Source: CAD feature listing. Evaluate the final solid. Frame: model axes, mm. Face numbers are marked on the shaded views. Give positions to 0.01 mm unless a question says otherwise; leave off trailing zeros. Loops run counter-clockwise (first coordinate to the right, second up) from the corner with the lowest first, then second, coordinate; pieces in that order, holes last.
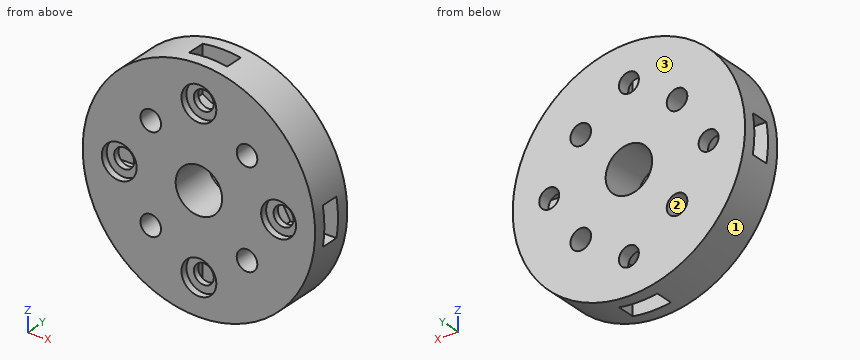
```python
from build123d import *

# Parameters (mm, degrees)
SKETCH1_R                      = 6.05
SKETCH1_R_2                    = 3.05
BOSS_EXTRUDE1_DEPTH            = 10
SKETCH2_R                      = 17.5
BOSS_EXTRUDE2_DEPTH            = 6.5
CUT_EXTRUDE1_REACH             = 28.693
SKETCH3_R                      = 1.5
CUT_EXTRUDE2_DEPTH             = 30.744747435
CUT_EXTRUDE2_DEPTH_BACK        = 30.744747435
SKETCH4_R                      = 1.5
CUT_EXTRUDE3_REACH             = 28.693
SKETCH6_R                      = 3.5
CUT_EXTRUDE3_DIRECTION_2_REACH = 28.693
SKETCH8_W                      = 5.75
SKETCH8_H                      = 2.75
CUT_EXTRUDE4_DEPTH             = 5
CUT_EXTRUDE5_DEPTH             = 2.75
CIRPATTERN1_START              = 11.875
CIRPATTERN1_OUTLINE_R          = 1.5
CIRPATTERN1_DEPTH              = 2.75
SKETCH10_R                     = 6.05
CUT_EXTRUDE6_DEPTH             = 10
SKETCH11_R                     = 1.55
CUT_EXTRUDE7_DEPTH             = 10
SKETCH12_R                     = 2.625
CUT_EXTRUDE8_DEPTH             = 1
CIRPATTERN2_COUNT              = 4


# Read off the part's stored shape, not the designer's step: CirPattern1
with BuildPart() as part:
    # Sketch1 → Boss-Extrude1 (new body)
    with BuildSketch(Plane(origin=(0, 0, 0), x_dir=(1, 0, 0), z_dir=(0, 1, 0))):
        with Locations(Location((0, 0, 0), (0, 0, 270))):
            Circle(SKETCH1_R)
        with Locations(Location((0, 0, 0), (0, 0, 270))):
            Circle(SKETCH1_R_2, mode=Mode.SUBTRACT)
    extrude(amount=BOSS_EXTRUDE1_DEPTH)

    # Sketch2 → Boss-Extrude2 (add)
    with BuildSketch(Plane(origin=(0, 10, 0), x_dir=(1, 0, 0), z_dir=(0, 1, 0))):
        with Locations(Location((0, 0, 0), (0, 0, 90))):
            Circle(SKETCH2_R)
    extrude(amount=BOSS_EXTRUDE2_DEPTH)

    # Sketch3 → Cut-Extrude1 (cut, up to next)
    with BuildSketch(Plane.XZ.offset(-10), mode=Mode.PRIVATE) as cut_extrude1_sk1:
        with Locations(Location((12, 0, 0), (0, 0, 270))):
            Circle(SKETCH3_R)
    cut_extrude1_tool1 = extrude(cut_extrude1_sk1.sketch, amount=-CUT_EXTRUDE1_REACH, mode=Mode.PRIVATE) & part.part
    # Sketch3 → Cut-Extrude1 (cut, up to next)
    with BuildSketch(Plane.XZ.offset(-10), mode=Mode.PRIVATE) as cut_extrude1_sk2:
        with Locations(Location((0, -12, 0), (0, 0, 270))):
            Circle(SKETCH3_R)
    cut_extrude1_tool2 = extrude(cut_extrude1_sk2.sketch, amount=-CUT_EXTRUDE1_REACH, mode=Mode.PRIVATE) & part.part
    # Sketch3 → Cut-Extrude1 (cut, up to next)
    with BuildSketch(Plane.XZ.offset(-10), mode=Mode.PRIVATE) as cut_extrude1_sk3:
        with Locations(Location((-12, 0, 0), (0, 0, 270))):
            Circle(SKETCH3_R)
    cut_extrude1_tool3 = extrude(cut_extrude1_sk3.sketch, amount=-CUT_EXTRUDE1_REACH, mode=Mode.PRIVATE) & part.part
    # Sketch3 → Cut-Extrude1 (cut, up to next)
    with BuildSketch(Plane.XZ.offset(-10), mode=Mode.PRIVATE) as cut_extrude1_sk4:
        with Locations(Location((0, 12, 0), (0, 0, 270))):
            Circle(SKETCH3_R)
    cut_extrude1_tool4 = extrude(cut_extrude1_sk4.sketch, amount=-CUT_EXTRUDE1_REACH, mode=Mode.PRIVATE) & part.part
    add(cut_extrude1_tool1.solids().sort_by_distance((12, 10, 0))[0], mode=Mode.SUBTRACT)
    add(cut_extrude1_tool2.solids().sort_by_distance((0, 10, -12))[0], mode=Mode.SUBTRACT)
    add(cut_extrude1_tool3.solids().sort_by_distance((-12, 10, 0))[0], mode=Mode.SUBTRACT)
    add(cut_extrude1_tool4.solids().sort_by_distance((0, 10, 12))[0], mode=Mode.SUBTRACT)

    # Sketch4 → Cut-Extrude2 (cut, two sides: drawn at the far end of the back side and taken through both)
    with BuildSketch(Plane.XY.offset(-CUT_EXTRUDE2_DEPTH_BACK)):
        with Locations((0, 4.916404418)):
            Circle(SKETCH4_R)
    extrude(amount=CUT_EXTRUDE2_DEPTH + CUT_EXTRUDE2_DEPTH_BACK, mode=Mode.SUBTRACT)

    # Sketch6 → Cut-Extrude3 (cut, up to next)
    with BuildSketch(Plane(origin=(0, 10, 0), x_dir=(-1, 0, 0), z_dir=(0, -1, 0)), mode=Mode.PRIVATE) as cut_extrude3_sk1:
        with Locations(Location((0, 0, 0), (0, 0, 270))):
            Circle(SKETCH6_R)
    cut_extrude3_tool1 = extrude(cut_extrude3_sk1.sketch, amount=-CUT_EXTRUDE3_REACH, mode=Mode.PRIVATE) & part.part
    add(cut_extrude3_tool1.solids().sort_by_distance((0, 10, 0))[0], mode=Mode.SUBTRACT)

    # Sketch6 → Cut-Extrude3 direction 2 (cut, up to next)
    with BuildSketch(Plane(origin=(0, 10, 0), x_dir=(-1, 0, 0), z_dir=(0, -1, 0)), mode=Mode.PRIVATE) as cut_extrude3_direction_2_sk1:
        with Locations(Location((0, 0, 0), (0, 0, 270))):
            Circle(SKETCH6_R)
    cut_extrude3_direction_2_tool1 = extrude(cut_extrude3_direction_2_sk1.sketch, amount=CUT_EXTRUDE3_DIRECTION_2_REACH, mode=Mode.PRIVATE) & part.part
    add(cut_extrude3_direction_2_tool1.solids().sort_by_distance((0, 10, 0))[0], mode=Mode.SUBTRACT)

    # Sketch8 → Cut-Extrude4 (cut)
    with BuildSketch(Plane(origin=(17.5, 0, 0), x_dir=(0, 0, -1), z_dir=(1, 0, 0))):
        with Locations((0, 13.25)):
            Rectangle(SKETCH8_W, SKETCH8_H)
    extrude(amount=-CUT_EXTRUDE4_DEPTH, mode=Mode.SUBTRACT)

    # Sketch9 → Cut-Extrude5 (cut)
    with BuildSketch(Plane.XZ.offset(-14.625)):
        Polygon((15.319764048, 0), (13.659882024, 2.875), (10.340117976, 2.875), (8.680235952, 0), (10.340117976, -2.875), (13.659882024, -2.875), align=None)
    extrude(amount=CUT_EXTRUDE5_DEPTH, mode=Mode.SUBTRACT)

    # CirPattern1 outline → CirPattern1 (cut)
    # profile 1 of 3: a face of its own
    with BuildSketch(Plane(origin=(0, 0, 0), x_dir=(1, 0, 0), z_dir=(0, 1, 0)).offset(CIRPATTERN1_START)):
        with BuildLine():
            Line((-8.680235952, 0), (-10.340117976, 2.875))
            Line((-10.340117976, 2.875), (-17.26222393, 2.875))
            ThreePointArc((-17.26222393, 2.875), (-17.5, 0), (-17.26222393, -2.875))
            Line((-17.26222393, -2.875), (-10.340117976, -2.875))
            Line((-10.340117976, -2.875), (-8.680235952, 0))
        make_face()
        with Locations((-12, 0)):
            Circle(CIRPATTERN1_OUTLINE_R, mode=Mode.SUBTRACT)
    # profile 2 of 3: a face of its own
    with BuildSketch(Plane(origin=(0, 0, 0), x_dir=(1, 0, 0), z_dir=(0, 1, 0)).offset(CIRPATTERN1_START)):
        with BuildLine():
            ThreePointArc((2.875, 17.26222393), (0, 17.5), (-2.875, 17.26222393))
            Line((-2.875, 17.26222393), (-2.875, 10.340117976))
            Line((-2.875, 10.340117976), (0, 8.680235952))
            Line((0, 8.680235952), (2.875, 10.340117976))
            Line((2.875, 10.340117976), (2.875, 17.26222393))
        make_face()
        with Locations((0, 12)):
            Circle(CIRPATTERN1_OUTLINE_R, mode=Mode.SUBTRACT)
    # profile 3 of 3: a face of its own
    with BuildSketch(Plane(origin=(0, 0, 0), x_dir=(1, 0, 0), z_dir=(0, 1, 0)).offset(CIRPATTERN1_START)):
        with BuildLine():
            Line((-2.875, -10.340117976), (-2.875, -17.26222393))
            ThreePointArc((-2.875, -17.26222393), (0, -17.5), (2.875, -17.26222393))
            Line((2.875, -17.26222393), (2.875, -10.340117976))
            Line((2.875, -10.340117976), (0, -8.680235952))
            Line((0, -8.680235952), (-2.875, -10.340117976))
        make_face()
        with Locations((0, -12)):
            Circle(CIRPATTERN1_OUTLINE_R, mode=Mode.SUBTRACT)
    extrude(amount=CIRPATTERN1_DEPTH, mode=Mode.SUBTRACT)

    # Sketch10 → Cut-Extrude6 (cut)
    with BuildSketch(Plane.XZ):
        Circle(SKETCH10_R)
    extrude(amount=-CUT_EXTRUDE6_DEPTH, mode=Mode.SUBTRACT)

    # Sketch11 → Cut-Extrude7 (cut)
    with BuildSketch(Plane(origin=(0, 16.5, 0), x_dir=(1, 0, 0), z_dir=(0, 1, 0))):
        with Locations(Location((-7.247844507, -7.247844507, 0), (0, 0, 270))):
            Circle(SKETCH11_R)
        with Locations(Location((-7.247844507, 7.247844507, 0), (0, 0, 270))):
            Circle(SKETCH11_R)
        with Locations(Location((7.247844507, 7.247844507, 0), (0, 0, 270))):
            Circle(SKETCH11_R)
        with Locations(Location((7.247844507, -7.247844507, 0), (0, 0, 270))):
            Circle(SKETCH11_R)
    extrude(amount=-CUT_EXTRUDE7_DEPTH, mode=Mode.SUBTRACT)

    # Sketch12 → Cut-Extrude8 (cut)
    with BuildSketch(Plane.XZ.offset(-10)):
        with Locations(Location((0, -12, 0), (0, 0, 270))):
            Circle(SKETCH12_R)
    cut_extrude8 = extrude(amount=-CUT_EXTRUDE8_DEPTH, mode=Mode.SUBTRACT)

    # CirPattern2: Cut-Extrude8 ×4 about axis
    cirpattern2_axis = Axis((0, 0, 0), (0, 1, 0))
    for i in range(1, CIRPATTERN2_COUNT):
        add(cut_extrude8.rotate(cirpattern2_axis, i * 360 / CIRPATTERN2_COUNT), mode=Mode.SUBTRACT)


solid = part.part
```
(1) Section A-A, the plane z = -12. Return the cut outline in (x, y) (3 decimals).
A:
outline: (-12.738, 10) - (-2.625, 10) - (-2.625, 11) - (-1.5, 11) - (-1.5, 11.875) - (-2.875, 11.875) - (-2.875, 14.625) - (-1.5, 14.625) - (-1.5, 16.5) - (-12.738, 16.5) - close; (1.5, 11) - (2.625, 11) - (2.625, 10) - (12.738, 10) - (12.738, 16.5) - (1.5, 16.5) - (1.5, 14.625) - (2.875, 14.625) - (2.875, 11.875) - (1.5, 11.875) - close
(2) Section B-B, the plane x = 12. Return the cut outline in (y, z) (3 decimals), then the cut area to 3 significant figures.
A:
outline: (10, -12.738) - (16.5, -12.738) - (16.5, -1.5) - (14.625, -1.5) - (14.625, -2.875) - (11.875, -2.875) - (11.875, -1.5) - (11, -1.5) - (11, -2.625) - (10, -2.625) - close; (10, 2.625) - (11, 2.625) - (11, 1.5) - (11.875, 1.5) - (11.875, 2.875) - (14.625, 2.875) - (14.625, 1.5) - (16.5, 1.5) - (16.5, 12.738) - (10, 12.738) - close
area: 136 mm2
(3) Ray query, line 1 along X through (y, z) = (15.3, 0); line 2 along Z through (x, y) = (8.5, 10.75); line 3 along X through (y, z) = (12.75, -8). Return the intervals inside material, ascending.
A:
line 1: x = -17.5 to -13.5, -10.5 to -3.5, 3.5 to 10.5, 13.5 to 17.5
line 2: z = -15.3 to -8.16, -6.33 to 6.33, 8.16 to 15.3
line 3: x = -15.56 to -8.6, -5.89 to 5.89, 8.6 to 15.56
(4) First-contact query: pin 1 (3 mm diameter, centred on x = -12, y = 13.5, fed in from +Z); pin 2 (2.5 mm diameter, centred on x = -12, z = 0, fed in from +Y); pin 3 (3 mm diameter, centred on y = 13.5, z = 14.5, fed in from -X); pin 4 (3 mm diameter, centred on y = 11, z = 8.5, fed in from +X). Flat tips, straight axial feed; report the tip coordinate or a pass-through.
A:
pin 1: stops at z = 14
pin 2: passes through
pin 3: stops at x = -11.72
pin 4: stops at x = 16.04
(5) Section C-C, the plane y = 10.5. Count the separate pieces of the cut face and the enclosed holes in it, then the cut area to 3 significant figures.
A:
separate pieces: 1
enclosed holes: 9
area: 807 mm2
(6) Section D-D, the plane y = 12.75. Return the cut outline in (x, z) (3 decimals), then the cut area to 3 significant figures.
A:
outline: (-17.262, -2.875) arc R17.5 ccw to (-2.875, -17.262) - (-2.875, -10.34) - (0, -8.68) - (2.875, -10.34) - (2.875, -17.262) arc R17.5 ccw to (17.262, -2.875) - (10.34, -2.875) - (8.68, 0) - (10.34, 2.875) - (17.262, 2.875) arc R17.5 ccw to (2.875, 17.262) - (2.875, 10.34) - (0, 8.68) - (-2.875, 10.34) - (-2.875, 17.262) arc R17.5 ccw to (-17.262, 2.875) - (-10.34, 2.875) - (-8.68, 0) - (-10.34, -2.875) - close; hole circle Ø3.1 at (-7.248, -7.248); hole circle Ø3.1 at (-7.248, 7.248); hole circle Ø7 at (0, 0); hole circle Ø3.1 at (7.248, -7.248); hole circle Ø3.1 at (7.248, 7.248)
area: 711 mm2
(7) Mould query, pull axis X, two halves, no side actions, for the marked faces 1, 2 and 3. Classes: pulls with the +X half, pulls with the -X half, needs draft (parallel to the pull), parting line crosses it, or undercut.
A:
face 1: parting line crosses it
face 2: undercut
face 3: needs draft
